Read the model definition and answer for the solid it produces. Units are mm, in the model's axes. A direction names the side the tool comes from. Round coordinates to 2 decimals unless told otherwise and drop trailing zeros. Order: outer loops, then holes, each group sorted by start corner. A loop starts at its lowest first (then second) coordinate and runs counter-clockwise, first axis right, second up. Notation, with made-up numbers: (5.25, 78.25) -> (25.25, 78.25) arc R32 ccw to (25.25, 106.25) -> close; hole circle Ø1 at (39, -9.75). An arc over 180 degrees is marked (long way). Answer as a JSON object with one key per item and string values. Group by question number.
Item 1: Section C-C, the plane y = 22.5 is taken. Write down the section's boundary in (x, z).
Item 2: Section A-A, the plane z = 29 is taken. Write down the section's boundary in (x, y), plus the area to 3 significant figures.
Item 3: For faces 4 (the flat face through (-95.242, 10, 34)), 5 (the cylindrical face through (-27.5, 2.5, 32.8)), 6 (the cylindrical face through (-100.25, 11.95, 33.93)), determine the directions among +Z, -Z, +X, -X, +Y, -Y from which every point of the face is accessible in a straight line to the end or side of a thin tool.
Item 4: Section B-B, the plane x = -40.5 is taken. Write down the section's boundary in (y, z).
Item 5: The mould has two halves that part along X. Classify faces 1 (the cylindrical face through (-101.34, 2.46, -32.31)), 2 (the flat face through (-64, 13, 37.33)), 3 (the flat face through (-64, 12, 38.33)): pulls with the +X half, pulls with the -X half, needs draft (parallel to the pull), parting line crosses it, or undercut.
Item 6: Consider probe 1 along Z at (x, y) = (-98.5, 17.5); probe 2 along X at (y, z) = (7.25, -17.5); probe 3 along Z at (x, y) = (-55.5, 13.5). Determine where each line is inside the solid, lowest interval first. Write a range as from..to.
Item 7: Given P1, Ø4.5, axis at x = -98.5, z = -31, coming from the +Y side; P2, Ø2.5, axis at x = -28.74, z = 35.09, coming from the +Y side; P3, Ø3, axis at x = -70.5, z = -19.5, coming from the +Y side, each flat-ended and moving along its own axis, determine where each tip first touches the part or whether it passes through.
Item 8: Section D-D, the plane z = -22 is taken. Write down the section's boundary in (x, y).
Autodesk Fusion 360 part; units mm, degrees
sketch "Sketch1" plane through (0, 0, 0) normal (0, 1, 0) x (1, 0, 0)
  arc A0 (-114.2414, 36.1703) -> (-116.2414, 34.1703) centre (-114.2414, 34.1703) ccw
  arc A1 (-114.2414, 36.1703) -> (-116.2414, 34.1703) centre (-114.2414, 34.1703) ccw
  arc A2 (-13.2414, -38.8297) -> (-11.2414, -36.8297) centre (-13.2414, -36.8297) ccw
  arc A3 (-116.2414, -36.8297) -> (-114.2414, -38.8297) centre (-114.2414, -36.8297) ccw
  arc A4 (-116.2414, -36.8297) -> (-114.2414, -38.8297) centre (-114.2414, -36.8297) ccw
  arc A5 (-13.2414, -38.8297) -> (-11.2414, -36.8297) centre (-13.2414, -36.8297) ccw
  circle A6 centre (-98.7415, -35.0863) radius 1.55
  circle A7 centre (-98.7415, 32.427) radius 1.55
  line L0 (-11.2414, -36.8297) -> (-11.2414, 34.1703)
  circle A8 centre (-28.7414, -35.0863) radius 1.55
  arc A9 (-11.2414, 34.1703) -> (-13.2414, 36.1703) centre (-13.2414, 34.1703) ccw
  arc A10 (-11.2414, 34.1703) -> (-13.2414, 36.1703) centre (-13.2414, 34.1703) ccw
  circle A11 centre (-28.7414, 32.427) radius 1.55
  line L1 (-116.2414, -36.8297) -> (-116.2414, 34.1703)
  line L2 (-13.2414, 36.1703) -> (-114.2414, 36.1703)
  line L3 (-114.2414, 36.1703) -> (-13.2414, 36.1703)
  line L4 (-114.2414, -38.8297) -> (-13.2414, -38.8297)
  line L5 (-116.2414, 34.1703) -> (-116.2414, -36.8297)
  line L6 (-11.2414, 34.1703) -> (-11.2414, -36.8297)
  line L7 (-13.2414, -38.8297) -> (-114.2414, -38.8297)
  line L8 (-12.7414, -36.8297) -> (-12.7414, 34.1703)
  arc A12 (-12.7414, 34.1703) -> (-13.2414, 34.6703) centre (-13.2414, 34.1703) ccw
  line L9 (-13.2414, 34.6703) -> (-114.2414, 34.6703)
  arc A13 (-114.2414, 34.6703) -> (-114.7414, 34.1703) centre (-114.2414, 34.1703) ccw
  line L10 (-114.7414, 34.1703) -> (-114.7414, -36.8297)
  arc A14 (-114.7414, -36.8297) -> (-114.2414, -37.3297) centre (-114.2414, -36.8297) ccw
  line L11 (-114.2414, -37.3297) -> (-13.2414, -37.3297)
  arc A15 (-13.2414, -37.3297) -> (-12.7414, -36.8297) centre (-13.2414, -36.8297) ccw
  circle A16 centre (-98.7415, -35.0863) radius 2.6
  circle A17 centre (-28.7414, -35.0863) radius 2.6
  circle A18 centre (-98.7415, 32.427) radius 2.6
  circle A19 centre (-28.7414, 32.427) radius 2.6
  circle A20 centre (-98.7415, -35.0863) radius 1.9
  circle A21 centre (-28.7414, -35.0863) radius 1.9
  circle A22 centre (-98.7415, 32.427) radius 1.9
  circle A23 centre (-28.7414, 32.427) radius 1.9
  line L12 (-11.7414, -36.8297) -> (-11.7414, 34.1703)
  arc A24 (-11.7414, 34.1703) -> (-13.2414, 35.6703) centre (-13.2414, 34.1703) ccw
  line L13 (-13.2414, 35.6703) -> (-114.2414, 35.6703)
  arc A25 (-114.2414, 35.6703) -> (-115.7414, 34.1703) centre (-114.2414, 34.1703) ccw
  line L14 (-115.7414, 34.1703) -> (-115.7414, -36.8297)
  arc A26 (-115.7414, -36.8297) -> (-114.2414, -38.3297) centre (-114.2414, -36.8297) ccw
  line L15 (-114.2414, -38.3297) -> (-13.2414, -38.3297)
  arc A27 (-13.2414, -38.3297) -> (-11.7414, -36.8297) centre (-13.2414, -36.8297) ccw
  line L16 (-38.2137, -26.6593) -> (-38.2137, -31.8593)
  line L17 (-38.7137, -32.3593) -> (-51.7137, -32.3593)
  arc A28 (-52.2137, -31.8593) -> (-51.7137, -32.3593) centre (-51.7137, -31.8593) ccw
  line L18 (-52.2137, -31.8593) -> (-52.2137, -26.6593)
  arc A29 (-38.2137, -26.6593) -> (-38.7137, -26.1593) centre (-38.7137, -26.6593) ccw
  line L19 (-51.7137, -26.1593) -> (-38.7137, -26.1593)
  arc A30 (-38.7137, -32.3593) -> (-38.2137, -31.8593) centre (-38.7137, -31.8593) ccw
  arc A31 (-51.7137, -26.1593) -> (-52.2137, -26.6593) centre (-51.7137, -26.6593) ccw
  point P0 (-38.2137, -32.3593)
  point P1 (-52.2137, -32.3593)
  point P2 (-52.2137, -26.1593)
  dimension "d1" = -1.5
  dimension "d16" = 5.2
  dimension "d17" = 5.2
  dimension "d18" = 5.2
  dimension "d19" = 5.2
  dimension "d22" = 3.8
  dimension "d23" = 3.8
  dimension "d24" = 3.8
  dimension "d25" = 3.8
  dimension "d28" = -0.5
  dimension "d31" = 6.2
  dimension "d32" = 14
  dimension "d33" = 0.5
  dimension "d34" = 0.5
  dimension "d35" = 0.5
extrude "Extrude1" add sketch "Sketch1" along normal blind 1.9 contours A0 A1 A2 A3 A4 A5 L0 A9 A10 L1 L2 L3 L4 L5 L6 L7 | L8 A12 L9 A13 L10 A14 L11 A15 A16 A17 A18 A19 | L11 A17 | L11 A17 | L9 A19 | L9 A19 | L11 A16 | L11 A16 | L9 A18 | L9 A18 | A20 | A21 | A22 | A23 | L12 A24 L13 A25 L14 A26 L15 A27 | L16 L17 A28 L18 A29 L19 A30 A31
extrude "Extrude2" add sketch "Sketch1" along normal blind 25 contours A0 A1 A2 A3 A4 A5 L0 A9 A10 L1 L2 L3 L4 L5 L6 L7 | L11 A17 | L9 A19 | L11 A16 | L9 A18 | L12 A24 L13 A25 L14 A26 L15 A27 picked at (-28.4059, -37.381) picked at (-28.6269, 34.8843) picked at (-98.406, -37.381) picked at (-98.9586, 34.8329)
sketch "Sketch2" plane through (0, 1.9, 0) normal (0, 1, 0) x (-1, 0, 0)
  line L0 (12.7414, 36.8297) -> (12.7414, -34.1703)
  arc A0 (12.7414, -34.1703) -> (13.2414, -34.6703) centre (13.2414, -34.1703) ccw
  line L1 (13.2414, -34.6703) -> (114.2414, -34.6703)
  arc A1 (114.2414, -34.6703) -> (114.7414, -34.1703) centre (114.2414, -34.1703) ccw
  line L2 (114.7414, -34.1703) -> (114.7414, 36.8297)
  arc A2 (114.7414, 36.8297) -> (114.2414, 37.3297) centre (114.2414, 36.8297) ccw
  line L3 (114.2414, 37.3297) -> (13.2414, 37.3297)
  arc A3 (13.2414, 37.3297) -> (12.7414, 36.8297) centre (13.2414, 36.8297) ccw
  circle A4 centre (98.7415, 35.0863) radius 1.55
  circle A5 centre (98.7415, -32.427) radius 1.55
  circle A6 centre (28.7414, -32.427) radius 1.55
  circle A7 centre (28.7414, 35.0863) radius 1.55
  line L4 (32.2414, 38.5863) -> (25.2414, 38.5863)
  line L5 (25.2414, 38.5863) -> (25.2414, 31.5863)
  line L6 (25.2414, 31.5863) -> (32.2414, 31.5863)
  line L7 (32.2414, 31.5863) -> (32.2414, 38.5863)
  line L8 (32.2414, 38.5863) -> (25.2414, 31.5863) construction
  line L9 (25.2414, 38.5863) -> (32.2414, 31.5863) construction
  line L10 (102.2415, 38.5863) -> (95.2415, 38.5863)
  line L11 (95.2415, 38.5863) -> (95.2415, 31.5863)
  line L12 (95.2415, 31.5863) -> (102.2415, 31.5863)
  line L13 (102.2415, 31.5863) -> (102.2415, 38.5863)
  line L14 (102.2415, 38.5863) -> (95.2415, 31.5863) construction
  line L15 (95.2415, 38.5863) -> (102.2415, 31.5863) construction
  line L16 (32.2414, -28.927) -> (25.2414, -28.927)
  line L17 (25.2414, -28.927) -> (25.2414, -35.927)
  line L18 (25.2414, -35.927) -> (32.2414, -35.927)
  line L19 (32.2414, -35.927) -> (32.2414, -28.927)
  line L20 (32.2414, -28.927) -> (25.2414, -35.927) construction
  line L21 (25.2414, -28.927) -> (32.2414, -35.927) construction
  line L22 (102.2415, -28.927) -> (95.2415, -28.927)
  line L23 (95.2415, -28.927) -> (95.2415, -35.927)
  line L24 (95.2415, -35.927) -> (102.2415, -35.927)
  line L25 (102.2415, -35.927) -> (102.2415, -28.927)
  line L26 (102.2415, -28.927) -> (95.2415, -35.927) construction
  line L27 (95.2415, -28.927) -> (102.2415, -35.927) construction
  point P0 (28.7414, 35.0863)
  point P1 (98.7415, 35.0863)
  point P2 (28.7414, -32.427)
  point P3 (98.7415, -32.427)
  dimension "d6" = 7
  dimension "d7" = 7
  dimension "d8" = 7
  dimension "d9" = 7
  dimension "d10" = 7
  dimension "d11" = 7
  dimension "d12" = 7
  dimension "d13" = 7
extrude "Extrude3" add sketch "Sketch2" along normal blind 17.2 contours L3 L5 L6 L7 | L1 L16 L17 L19 | L3 L11 L12 L13 | L1 L22 L23 L25
extrude "Extrude4" cut sketch "Sketch1" along normal blind 5 contours L11 A17 | L11 A17 | L9 A19 | L9 A19 | L11 A16 | L11 A16 | L9 A18 | L9 A18 | A20 | A21 | A22 | A23
extrude "Extrude5" cut sketch "Sketch1" along normal blind 38 contours A20 | A21 | A22 | A23
extrude "Extrude6" cut sketch "Sketch1" along normal blind 69 contours A0 A1 A2 A3 A4 A5 L0 A9 A10 L1 L2 L3 L4 L5 L6 L7
extrude "Extrude7" cut sketch "Sketch1" along normal blind 24 contours L16 L17 A28 L18 A29 L19 A30 A31
sketch "Sketch3" plane through (0, 0, 38.3297) normal (0, 0, 1) x (-1, 0, 0)
  line L0 (13.2414, -25) -> (114.2414, -25)
  line L1 (114.2414, -25) -> (114.2414, 0)
  line L2 (114.2414, 0) -> (13.2414, 0)
  line L3 (13.2414, 0) -> (13.2414, -25)
equation "d14 = 19.00 mm - 1.8 mm"
Values found:
{
 "1": {"outline": "(-115.74, -34.17) arc R1.5 ccw to (-114.24, -35.67) -> (-13.24, -35.67) arc R1.5 ccw to (-11.74, -34.17) -> (-11.74, 36.83) arc R1.5 ccw to (-13.24, 38.33) -> (-114.24, 38.33) arc R1.5 ccw to (-115.74, 36.83) -> close; hole (-114.74, -34.17) arc R0.5 ccw to (-114.24, -34.67) -> (-13.24, -34.67) arc R0.5 ccw to (-12.74, -34.17) -> (-12.74, 36.83) arc R0.5 ccw to (-13.24, 37.33) -> (-114.24, 37.33) arc R0.5 ccw to (-114.74, 36.83) -> close"},
 "2": {"outline": "(-115.74, 0) -> (-52.21, 0) -> (-52.21, 1.9) -> (-114.74, 1.9) -> (-114.74, 25) -> (-115.74, 25) -> close; (-38.21, 0) -> (-11.74, 0) -> (-11.74, 25) -> (-12.74, 25) -> (-12.74, 1.9) -> (-38.21, 1.9) -> close", "area": "217 mm2"},
 "3": {"face 4": "+Y", "face 5": "-Y", "face 6": "+Y, -Y"},
 "4": {"outline": "(0, -35.67) -> (25, -35.67) -> (25, -34.67) -> (1.9, -34.67) -> (1.9, 26.16) -> (0, 26.16) -> close; (0, 32.36) -> (1.9, 32.36) -> (1.9, 37.33) -> (25, 37.33) -> (25, 38.33) -> (0, 38.33) -> close"},
 "5": {"face 1": "undercut", "face 2": "undercut", "face 3": "needs draft"},
 "6": {"probe 1": "-35.67..-34.31, -30.54..-28.93, 31.59..33.2, 36.97..38.33", "probe 2": "-115.74..-114.74, -12.74..-11.74", "probe 3": "-35.67..-34.67, 37.33..38.33"},
 "7": {"P1": "y = 19.1", "P2": "through", "P3": "y = 1.9"},
 "8": {"outline": "(-115.74, 0) -> (-11.74, 0) -> (-11.74, 25) -> (-12.74, 25) -> (-12.74, 1.9) -> (-114.74, 1.9) -> (-114.74, 25) -> (-115.74, 25) -> close"}
}
